Part print with two shaded views. Sizes in mm from the minimum x, y, z corner. Coordinates: 2 decimals unless noted, no trailing zeros. Write each loop counter-clockwise with the first axis right and the second up, starting at its lowest first coordinate (ties: lowest second). Pieces come first, ordered by that corner, then holes.
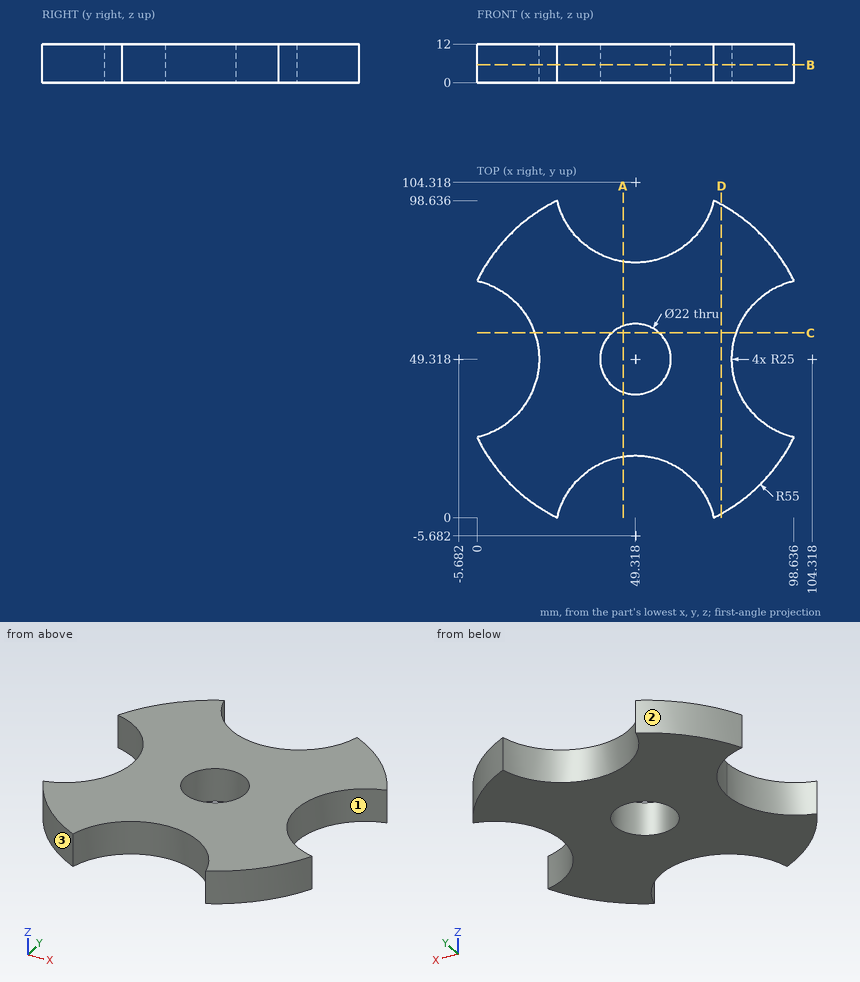
(1) Probe L1, parallel to X at y = 5, z = 8.5 (1 decimal); L2, parallel to Y at x = 88.5, z = 1.5 (1 decimal). List the from-to ranges inside material, lowest first.
(2) Slice it at B-B, the plane z = 5.5. List the corners of the cut face in (x, y), and give its area (3 significant figures).
(3) Two-plate mould, pull along Y, no slides. Class the marked faces 1, 2 and 3: pulls with the +Y half, pulls with the -Y half, needs draft (parallel to the pull), parting line crosses it, or undercut.
(4) Slice it at D-D, the plane x = 76. List the corners of the cut face in (y, z), and give its area (3 significant figures).
(5) Slice it at C-C, the plane y = 57.5. List the corners of the cut face in (x, z) (1 decimal).
(6) Flat gauge pins, fed straight in: P1, Ø3, axis at x = 38.5, z = 3, coming from the -Y side; P2, Ø20, axis at x = 49.32, y = 49.32, coming from the -Z side; P3, Ø1, axis at y = 51.5, z = 1.5, coming from the +X side. Where does each tip first touch, or does it go through?
(7) Slice it at A-A, the plane x = 45.5. List the corners of the cut face in (y, z) (1 decimal).
Results:
1. L1: x = 16.7 to 26.7, 71.9 to 81.9
1. L2: y = 10.7 to 30, 68.7 to 87.9
2. outline: (0, 24.97) arc R55 ccw to (24.97, 0) arc R25 cw to (73.66, 0) arc R55 ccw to (98.64, 24.97) arc R25 cw to (98.64, 73.66) arc R55 ccw to (73.66, 98.64) arc R25 cw to (24.97, 98.64) arc R55 ccw to (0, 73.66) arc R25 cw to (19.32, 49.32) arc R25 cw to start; hole circle Ø22 at (49.32, 49.32)
2. area: 5,580 mm2
3. face 1: undercut
3. face 2: pulls with the +Y half
3. face 3: pulls with the -Y half
4. outline: (1.22, 0) - (97.41, 0) - (97.41, 12) - (1.22, 12) - close
4. area: 1,150 mm2
5. outline: (17.9, 0) - (42, 0) - (42, 12) - (17.9, 12) - close; (56.7, 0) - (80.7, 0) - (80.7, 12) - (56.7, 12) - close
6. P1: stops at y = 16.07
6. P2: passes through
6. P3: stops at x = 79.46
7. outline: (19, 0) - (39, 0) - (39, 12) - (19, 12) - close; (59.6, 0) - (79.6, 0) - (79.6, 12) - (59.6, 12) - close
